Part print with two shaded views. Sizes in mm from the minimum x, y, z corner. A direction names the side the tool comes from. Give positions to 0.01 mm unless a question says otherwise; leave off trailing zeros. Order: outer loops, then holes, each group sorted by start corner. A loop starts at its lowest first (then second) coordinate and runs counter-clockwise, first axis right, second up. Notation, with made-up numbers: M 75,64.5 L 102,64.5 A20 ccw 102,80.5 Z; hole C 8.5,72.5 d9. An arc over 180 degrees is marked long. Answer as CSV lines item,"result".
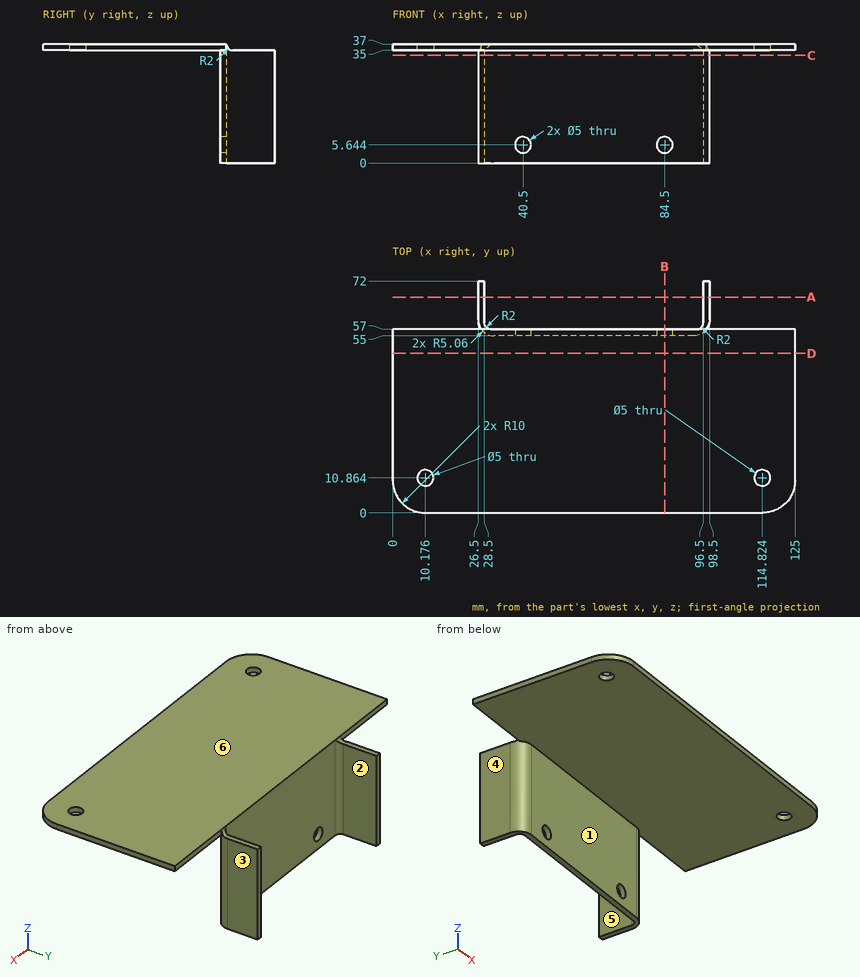
Item 1: Probe line 1 along X through (y, z) = (66, 29); line 2 along Z through (x, y) = (40.5, 56.5); line 3 along Y through (x, z) = (61.5, 5.5). List the from-to ranges inside material, lowest first. Write a range as from..to.
Geometry says:
line 1,"x = 26.5..28.5, 96.5..98.5"
line 2,"z = 0..3.14, 8.14..37"
line 3,"y = 55..57"
Item 2: Band-saw the part on D-D (y = 49.5). Give the cut face in (x, z).
Geometry says:
outline,"M 0,35 L 125,35 L 125,37 L 0,37 Z"
Item 3: Band-saw the part on C-C (z = 33.5). Give the cut face in (x, y), and give its area (3 significant figures).
Geometry says:
outline,"M 26.5,60.06 A5.06 ccw 31.56,55 L 93.44,55 A5.06 ccw 98.5,60.06 L 98.5,72 L 96.5,72 L 96.5,59 A2 cw 94.5,57 L 30.5,57 A2 cw 28.5,59 L 28.5,72 L 26.5,72 Z"
area,"195 mm2"
Item 4: Pull direction X, two halves, no side cores. Call the marked faces 3, 4, 5 and 6: released by +X, released by -X, zero draft, split by the parting line, or undercut.
Geometry says:
face 3,"released by +X"
face 4,"released by -X"
face 5,"undercut"
face 6,"zero draft"
Item 5: 3-axis set-ups, long thin cutter, end or side, ignore diameter. For the marked faces 1 and 2: which of +Z, -Z, +X, -X, +Y, -Y reach the whole face in a straight line?
Geometry says:
face 1,"-Z, +X, -X, -Y"
face 2,"+Z, -Z, +Y"
Item 6: Drop flat-ended pins along their axis: pin 1 (1 mm diameter, centred on x = 44.5, z = 29.5, fed in from -Y); pin 2 (3 mm diameter, centred on x = 114.82, y = 10.86, fed in from -Z); pin 3 (2 mm diameter, centred on x = 64, z = 14.5, fed in from +Y); pin 4 (3 mm diameter, centred on y = 56, z = 4.5, fed in from +X) (1 decimal). Give the stop position or say it passes through.
Geometry says:
pin 1,"stops at y = 55"
pin 2,"passes through"
pin 3,"stops at y = 57"
pin 4,"stops at x = 97.8"
Item 7: Band-saw the part on B-B (x = 84.5). Give the cut face in (y, z).
Geometry says:
outline,"M 0,35 L 55,35 L 55,8.14 L 57,8.14 L 57,37 L 0,37 Z; M 55,0 L 57,0 L 57,3.14 L 55,3.14 Z"
Item 8: Band-saw the part on A-A (y = 67). Give the cut face in (x, z).
Geometry says:
outline,"M 26.5,0 L 28.5,0 L 28.5,35 L 26.5,35 Z; M 96.5,0 L 98.5,0 L 98.5,35 L 96.5,35 Z"
